Autodesk Inventor part; units mm, degrees
ref_plane "YZ Plane" through (0, 0, 0) normal (1, 0, 0) x (0, 1, 0)
ref_plane "XZ Plane" through (0, 0, 0) normal (0, 1, 0) x (-1, 0, 0)
ref_plane "XY Plane" through (0, 0, 0) normal (0, 0, 1) x (1, 0, 0)
sketch "Sketch1" plane through (0, 0, 0) normal (0, 0, 1) x (1, 0, 0)
  line L0 (0, 0) -> (0.9125, 0)
  line L1 (0.9125, 0) -> (0.9125, -6.731)
  line L2 (0.9125, -6.731) -> (5.9125, -6.731)
  line L3 (5.9125, -6.731) -> (5.9125, 0)
  line L4 (5.9125, 0) -> (6.825, 0)
  line L5 (6.825, 0) -> (6.825, 13.269)
  line L6 (6.825, 13.269) -> (5.9125, 13.269)
  line L7 (5.9125, 13.269) -> (5.9125, 20)
  line L8 (5.9125, 20) -> (0.9125, 20)
  line L9 (0.9125, 20) -> (0.9125, 13.269)
  line L10 (0.9125, 13.269) -> (0, 13.269)
  line L11 (0, 13.269) -> (0, 0)
  dimension "d0" = 5
  dimension "d1" = 13.269
  dimension "d2" = 6.731
  dimension "d3" = 6.825
extrude "Extrusion1" add sketch "Sketch1" along normal blind 6.731
sketch "Sketch3" plane through (0, 0, 0) normal (0, 0, -1) x (-1, 0, 0)
  line L0 (0, 0) -> (-0.9125, 0)
  line L1 (-0.9125, 13.269) -> (0, 13.269)
  line L2 (-0.9125, 20) -> (-0.9125, 13.269)
  line L3 (-5.9125, 13.269) -> (-5.9125, 20)
  line L4 (-6.825, 13.269) -> (-5.9125, 13.269)
  line L5 (-5.9125, 0) -> (-6.825, 0)
  line L6 (-5.9125, -6.731) -> (-5.9125, 0)
  line L7 (-0.9125, 0) -> (-0.9125, -6.731)
  arc A0 (-0.9125, 0) -> (-0.9125, -3.176) centre (-0.9125, -1.588) ccw
  arc A1 (-5.9125, -3.176) -> (-5.9125, 0) centre (-5.9125, -1.588) ccw
  arc A2 (-5.9125, 13.269) -> (-5.9125, 16.445) centre (-5.9125, 14.857) ccw
  arc A3 (-0.9125, 16.445) -> (-0.9125, 13.269) centre (-0.9125, 14.857) ccw
  dimension "d13" = 1.588
extrude "Extrusion3" cut sketch "Sketch3" against normal up to next
equation "\"d2\" = THICKB"
equation "\"d4\" = THICKB"
equation "\"THICKA\" = 3.175"
equation "\"THICKB\" = 6.731"
equation "\"THICKC\" = 12.7"
equation "\"THICKPLY\" = 5"
equation "\"MAGDIA\" = 9.5"
equation "\"BALLDIA\" = 12"
properties part number "Carriage_Joint_Boltblock_Brace"
Input: part model. Units: mm. Frame: model coordinates. A direction names the side the tool comes from. Coordinates: 2 decimals unless noted, no trailing zeros. Order: outer loops, then holes, each group sorted by start corner. A loop starts at its lowest first (then second) coordinate and runs counter-clockwise, first axis right, second up. Notation, with made-up numbers: (-35.5, 15.25) - (13.5, 15.25) arc R29 cw to (13.5, 39.25) - close; hole circle Ø2 at (-2, 80). An arc over 180 degrees is marked (long way). Return JSON: item names as keys, results as strings.
Q1. Ray query, probe 1 along Y at (x, z) = (5.5, 2.5); probe 2 along Y at (x, z) = (5, 1); probe 3 along Y at (x, z) = (0.5, 5.75). Return the intervals inside material, ascending.
The answers:
{"probe 1": "y = -6.73 to -3.12, -0.05 to 13.32, 16.39 to 20", "probe 2": "y = -6.73 to -2.89, -0.29 to 13.56, 16.16 to 20", "probe 3": "y = 0 to 13.27"}
Q2. First-contact query: pin 1 (3 mm diameter, centred on x = 5, y = 7.5, fed in from -Z); pin 2 (1 mm diameter, centred on x = 6.5, z = 4, fed in from -Y); pin 3 (0.7 mm diameter, centred on x = 0.5, z = 2.5, fed in from +Y); pin 4 (3 mm diameter, centred on y = 18.5, z = 3.5, fed in from -X). Flat tips, straight axial feed; report the tip coordinate or a pass-through.
The answers:
{"pin 1": "stops at z = 0", "pin 2": "stops at y = 0", "pin 3": "stops at y = 13.27", "pin 4": "stops at x = 0.91"}
Q3. Cut plane A-A (x = 2). Return loops of the section in (y, z), then the cut area to 3 significant figures.
The answers:
{"outline": "(-6.73, 0) - (-2.75, 0) - (-2.75, 6.73) - (-6.73, 6.73) - close; (-0.43, 0) - (13.7, 0) - (13.7, 6.73) - (-0.43, 6.73) - close; (16.01, 0) - (20, 0) - (20, 6.73) - (16.01, 6.73) - close", "area": "149 mm2"}
Q4. Cut plane B-B (z = 1.25). Return loops of the section in (x, y) (1 decimal), then the cut area to 3 significant figures.
The answers:
{"outline": "(0, 0) - (0.9, 0) arc R1.6 cw to (0.9, -3.2) - (0.9, -6.7) - (5.9, -6.7) - (5.9, -3.2) arc R1.6 cw to (5.9, 0) - (6.8, 0) - (6.8, 13.3) - (5.9, 13.3) arc R1.6 cw to (5.9, 16.4) - (5.9, 20) - (0.9, 20) - (0.9, 16.4) arc R1.6 cw to (0.9, 13.3) - (0, 13.3) - close", "area": "142 mm2"}
Q5. Cut plane D-D (y = 14.5). Return loops of the section in (x, z), then the cut area to 3 significant figures.
The answers:
{"outline": "(2.46, 0) - (4.37, 0) - (4.37, 6.73) - (2.46, 6.73) - close", "area": "12.8 mm2"}
Q6. Cut plane C-C (x = 5). Return loops of the section in (y, z), then the cut area to 3 significant figures.
The answers:
{"outline": "(-6.73, 0) - (-2.89, 0) - (-2.89, 6.73) - (-6.73, 6.73) - close; (-0.29, 0) - (13.56, 0) - (13.56, 6.73) - (-0.29, 6.73) - close; (16.16, 0) - (20, 0) - (20, 6.73) - (16.16, 6.73) - close", "area": "145 mm2"}
Q7. Access query for faces 1 (the flat face through (0.912, -5, 3)), 2 (the flat face through (0.5, 13.269, 3.3)), 3 (the flat face through (6.4, 0, 3.3)), 4 (the flat face through (5.912, 18, 3)). Directions: +Z, -Z, +X, -X, +Y, -Y. A direction counts if a zero-diameter tool reaches every point of the face in a straight line with its end or side. Return the directions, or none.
The answers:
{"face 1": "+Z, -Z, -X, -Y", "face 2": "+Z, -Z, -X, +Y", "face 3": "+Z, -Z, +X, -Y", "face 4": "+Z, -Z, +X, +Y"}
